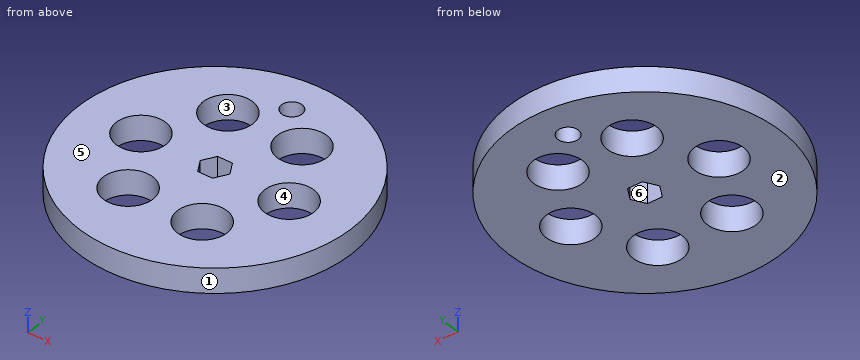
Autodesk Inventor part; units mm, degrees
ref_plane "YZ Plane" through (0, 0, 0) normal (1, 0, 0) x (0, 1, 0)
ref_plane "XZ Plane" through (0, 0, 0) normal (0, 1, 0) x (-1, 0, 0)
ref_plane "XY Plane" through (0, 0, 0) normal (0, 0, 1) x (1, 0, 0)
sketch "Sketch1" plane through (0, 0, 0) normal (0, 0, 1) x (1, 0, 0)
  circle A0 centre (0, 0) radius 69.85
  line L0 (7.6256, 0) -> (3.8128, -6.604)
  line L1 (3.8128, -6.604) -> (-3.8128, -6.604)
  line L2 (-3.8128, -6.604) -> (-7.6256, 0)
  line L3 (-7.6256, 0) -> (-3.8128, 6.604)
  line L4 (-3.8128, 6.604) -> (3.8128, 6.604)
  line L5 (3.8128, 6.604) -> (7.6256, 0)
  circle A1 centre (0, 50.8) radius 5.2705
  dimension "d0" = 139.7
  dimension "d1" = 13.208
  dimension "d2" = 10.541
  dimension "d5" = 50.8
extrude "Extrusion1" add sketch "Sketch1" along normal mid plane 12.7
sketch "Sketch2" plane through (0, 0, 6.35) normal (0, 0, 1) x (1, 0, 0)
  circle A0 centre (-38.1, 0) radius 12.7
  circle A1 centre (-19.05, -32.9956) radius 12.7
  circle A2 centre (19.05, -32.9956) radius 12.7
  circle A3 centre (38.1, 0) radius 12.7
  circle A4 centre (19.05, 32.9956) radius 12.7
  circle A5 centre (-19.05, 32.9956) radius 12.7
  point P0 (0, 0)
  dimension "d6" = 25.4
  dimension "d7" = 38.1
  dimension "d10" = 360
extrude "Extrusion2" cut sketch "Sketch2" against normal through all
properties part number "driveForPiston-4-in"
Model file for the job. Use its own axes, mm. Face numbers are marked on the shaded views. A direction names the side the tool comes from. Give positions to 0.01 mm unless a question says otherwise; leave off trailing zeros. Order: outer loops, then holes, each group sorted by start corner. A loop starts at its lowest first (then second) coordinate and runs counter-clockwise, first axis right, second up. Notation, with made-up numbers: (0.25, 67) - (37.25, 67) arc R19 ccw to (37.25, 78) - close; hole circle Ø11 at (83, -20.5). An arc over 180 degrees is marked (long way). Return JSON: item names as keys, results as strings.
1) Flat gauge pins, fed straight in: P1, Ø1.5, axis at y = 32, z = 2.5, coming from the +X side; P2, Ø1.5, axis at y = -6, z = 4, coming from the +X side; P3, Ø6, axis at x = -1.5, z = -3, coming from the +Y side. Where does each tip first touch, or does it go through?
Geometry says:
{"P1": "x = 62.47", "P2": "x = 69.65", "P3": "y = 69.85"}
2) Pull direction X, two halves, no side cores. Call the marked faces 1, 2, 3 and 4: pulls with the +X half, pulls with the -X half, needs draft (parallel to the pull), parting line crosses it, or undercut.
Geometry says:
{"face 1": "parting line crosses it", "face 2": "needs draft", "face 3": "undercut", "face 4": "undercut"}
3) 3-axis set-ups, long thin cutter, end or side, ignore diameter. For the marked faces 5 and 6: which of +Z, -Z, +X, -X, +Y, -Y reach the whole face in a straight line?
Geometry says:
{"face 5": "+Z, +X, -X, +Y, -Y", "face 6": "+Z, -Z"}
4) Cut at C-C, the plane z = -1.5. Count the separate pieces of the cut face and the enclosed holes in it, plus the area to 3 significant figures.
Geometry says:
{"separate pieces": "1", "enclosed holes": "8", "area": "12,000 mm²"}
5) Cut at B-B, the plane y = -9. Give the cut face in (x, z), plus the area to 3 significant figures.
Geometry says:
{"outline": "(-69.27, -6.35) - (-47.06, -6.35) - (-47.06, 6.35) - (-69.27, 6.35) - close; (-29.14, -6.35) - (29.14, -6.35) - (29.14, 6.35) - (-29.14, 6.35) - close; (47.06, -6.35) - (69.27, -6.35) - (69.27, 6.35) - (47.06, 6.35) - close", "area": "1,300 mm²"}
6) Cut at D-D, the plane y = 48.5. Give the cut face in (x, z).
Geometry says:
{"outline": "(-50.27, -6.35) - (-4.74, -6.35) - (-4.74, 6.35) - (-50.27, 6.35) - close; (4.74, -6.35) - (50.27, -6.35) - (50.27, 6.35) - (4.74, 6.35) - close"}
7) Cut at A-A, the plane x = 0. Give the cut face in (y, z), plus the area to 3 significant figures.
Geometry says:
{"outline": "(-69.85, -6.35) - (-6.6, -6.35) - (-6.6, 6.35) - (-69.85, 6.35) - close; (6.6, -6.35) - (45.53, -6.35) - (45.53, 6.35) - (6.6, 6.35) - close; (56.07, -6.35) - (69.85, -6.35) - (69.85, 6.35) - (56.07, 6.35) - close", "area": "1,470 mm²"}
8) Probe line 1 (Y direction, x = 0, z = -2.25); line 2 (Y direction, x = -20, z = -0.75); line 3 (X direction, y = 33, z = -5). List the from-to ranges inside material, lowest first. Write a range as from..to.
Geometry says:
{"line 1": "-69.85..-6.6, 6.6..45.53, 56.07..69.85", "line 2": "-66.93..-45.66, -20.33..20.33, 45.66..66.93", "line 3": "-61.56..-31.75, -6.35..6.35, 31.75..61.56"}
